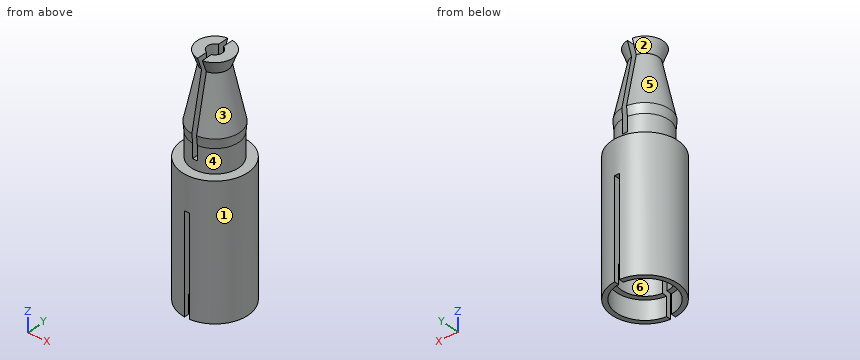
```python
from build123d import *

# Parameters (mm, degrees)
SKETCH001_R          = 2.47
POCKET_DEPTH         = 12
SKETCH002_R          = 0.7874
POCKET001_DEPTH      = 24.501
SKETCH003_R          = 3
POCKET002_DEPTH      = 2
SKETCH004_W          = 0.5
SKETCH004_H          = 15
SKETCH004_H_2        = 13
POCKET003_DEPTH      = 5
POCKET003_DEPTH_BACK = -5


with BuildPart() as part:
    # Sketch → Revolution (revolve)
    with BuildSketch(Plane.XZ):
        Polygon((2.5, 0), (3.5, 0), (3.5, -14), (0, -14), (0, 0), (0, 10.5), (1.9, 10.5), (1.4, 9.15), (2.6, 3.5), (2.5, 2.5), align=None)
    revolve(axis=Axis((0, 0, 0), (0, 0, 1)))

    # Sketch001 (on Face5 of Revolution) → Pocket (cut)
    with BuildSketch(Plane(origin=(0, 0, -14), x_dir=(1, 0, 0), z_dir=(0, 0, -1))):
        Circle(SKETCH001_R)
    extrude(amount=-POCKET_DEPTH, mode=Mode.SUBTRACT)

    # Sketch002 (on Face6 of Pocket) → Pocket001 (cut, through all)
    with BuildSketch(Plane(origin=(0, 0, 10.5), x_dir=(-1, 0, 0), z_dir=(0, 0, 1))):
        Circle(SKETCH002_R)
    extrude(amount=-POCKET001_DEPTH, mode=Mode.SUBTRACT)

    # Sketch003 (on Face9 of Pocket001) → Pocket002 (cut)
    with BuildSketch(Plane(origin=(0, 0, -14), x_dir=(1, 0, 0), z_dir=(0, 0, -1))):
        Circle(SKETCH003_R)
    extrude(amount=-POCKET002_DEPTH, mode=Mode.SUBTRACT)

    # Sketch004 → Pocket003 (cut, two sides)
    with BuildSketch(Plane.XZ) as pocket003_sk:
        with Locations((0, 8.5)):
            Rectangle(SKETCH004_W, SKETCH004_H)
        with Locations((0, -10.1)):
            Rectangle(SKETCH004_W, SKETCH004_H_2)
    extrude(amount=-POCKET003_DEPTH, mode=Mode.SUBTRACT)
    extrude(pocket003_sk.sketch, amount=-POCKET003_DEPTH_BACK, mode=Mode.SUBTRACT)


solid = part.part
```
Work out the finished part from the listing and answer in its coordinate system (mm). Face numbers are marked on the shaded views. A direction names the side the tool comes from. Round coordinates to 2 decimals unless told otherwise and drop trailing zeros. Write each loop counter-clockwise with the first axis right and the second up, starting at its lowest first coordinate (ties: lowest second). Pieces come first, ordered by that corner, then holes.
1) Flat-ended cylindrical pins translate along their axes: P1, Ø3, axis at x = 0, y = 0, coming from the -Z side; P2, Ø1.1, axis at y = 3, z = -9.5, coming from the -X side; P3, Ø2, axis at y = 1.5, z = 6.5, coming from the -X side. Find the tip coordinate at first contact, or state that the pin passes through.
2) Which of the six approach directions +Z, -Z, +X, -X, +Y, -Y give full straight-line access (tool end or side, diameter ignored) to the marked faces 3, 4, 5 and 6?
3) Determine the mould class of the marked faces 1 and 2 for opening direction Z: pulls with the +Z half, pulls with the -Z half, needs draft (parallel to the pull), parting line crosses it, or undercut.
4) A cutting plane is placed at D-D on y = 3.25. Determine the outline of the cut face in (x, z).
5) A cutting plane is placed at C-C on x = 0. Determine the outline of the cut face in (y, z), and give its area (3 significant figures).
6) A cutting plane is placed at A-A on y = 0. Determine the outline of the cut face in (x, z), and give its area (3 significant figures).
7) Consider probe 1 along X at (y, z) = (0, -6.25); probe 2 along Z at (x, y) = (-2.5, 1); probe 3 along X at (y, z) = (-0.5, 2.5). Determine where each line is inside the solid, lowest interval first.
Entries:
1. P1: stops at z = -2
1. P2: stops at x = -2.5
1. P3: stops at x = -1.97
2. face 3: +X
2. face 4: none
2. face 5: -X
2. face 6: -Z
3. face 1: needs draft
3. face 2: undercut
4. outline: (-1.3, -14) - (-0.25, -14) - (-0.25, -3.6) - (0.25, -3.6) - (0.25, -14) - (1.3, -14) - (1.3, 0) - (-1.3, 0) - close
5. outline: (-3.5, -3.6) - (-2.47, -3.6) - (-2.47, -2) - (-0.79, -2) - (-0.79, 1) - (-2.5, 1) - (-2.5, 0) - (-3.5, 0) - close; (0.79, -2) - (2.47, -2) - (2.47, -3.6) - (3.5, -3.6) - (3.5, 0) - (2.5, 0) - (2.5, 1) - (0.79, 1) - close
5. area: 17.6 mm2
6. outline: (-3.5, -14) - (-3, -14) - (-3, -12) - (-2.47, -12) - (-2.47, -2) - (-0.79, -2) - (-0.79, 10.5) - (-1.9, 10.5) - (-1.4, 9.15) - (-2.6, 3.5) - (-2.5, 2.5) - (-2.5, 0) - (-3.5, 0) - close; (0.79, -2) - (2.47, -2) - (2.47, -12) - (3, -12) - (3, -14) - (3.5, -14) - (3.5, 0) - (2.5, 0) - (2.5, 2.5) - (2.6, 3.5) - (1.4, 9.15) - (1.9, 10.5) - (0.79, 10.5) - close
6. area: 61.6 mm2
7. probe 1: x = -3.5 to -2.47, 2.47 to 3.5
7. probe 2: z = -12 to 0
7. probe 3: x = -2.45 to -0.61, 0.61 to 2.45
